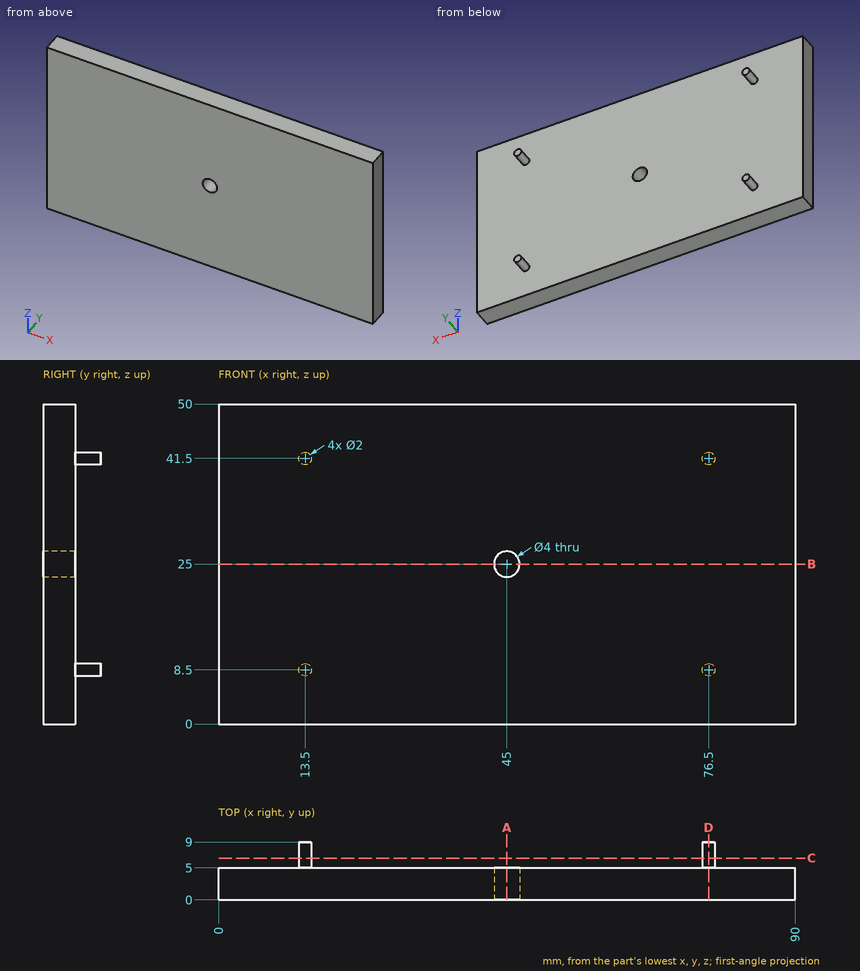
Print and shaded views of the part. All mm, measured from the part's lowest x, y and z. Coordinates: 2 decimals unless noted, no trailing zeros. Order: outer loops, then holes, each group sorted by start corner. A loop starts at its lowest first (then second) coordinate and runs counter-clockwise, first axis right, second up. Notation, with made-up numbers: M -22,80 L -1,80 A24 cw -1,93 Z; hole C -34.75,9.25 d11. An arc over 180 degrees is marked long. Answer as CSV lines item,"result".
1) Flat gauge pins, fed straight in: P1, Ø1, axis at x = 25.5, z = 26.5, coming from the -Y side; P2, Ø6.5, axis at x = 45, z = 25, coming from the +Y side. Where does each tip first touch, or does it go through?
Verdict:
P1,"y = 0"
P2,"y = 5"
2) Cut at C-C (y = 6.5). List the corners of the cut face in (x, z).
Verdict:
outline,"C 13.5,8.5 d2; C 13.5,41.5 d2; C 76.5,8.5 d2; C 76.5,41.5 d2"
3) Cut at A-A (x = 45). List the corners of the cut face in (y, z).
Verdict:
outline,"M 0,0 L 5,0 L 5,23 L 0,23 Z; M 0,27 L 5,27 L 5,50 L 0,50 Z"
4) Drill centre lines: L1, parallel to Z at x = 45, y = 3.15; L2, parallel to X at y = 2.65, z = 25; L3, parallel to Y at x = 52, z = 21.5. Where is each one in solid material? Low to high. Write a range as from..to.
Verdict:
L1,"0..23, 27..50"
L2,"0..43, 47..90"
L3,"0..5"
5) Cut at D-D (x = 76.5). List the corners of the cut face in (y, z).
Verdict:
outline,"M 0,0 L 5,0 L 5,7.5 L 9,7.5 L 9,9.5 L 5,9.5 L 5,40.5 L 9,40.5 L 9,42.5 L 5,42.5 L 5,50 L 0,50 Z"
6) Cut at B-B (z = 25). List the corners of the cut face in (x, y), then the cut area to 3 significant figures.
Verdict:
outline,"M 0,0 L 43,0 L 43,5 L 0,5 Z; M 47,0 L 90,0 L 90,5 L 47,5 Z"
area,"430 mm2"
